from build123d import *

# Parameters (mm, degrees)
F0_R     = 6.35
F1_DEPTH = 10.16
F2_R     = 6.3201010277
F3_DEPTH = 12.7
F5_DEPTH = 10.16
F6_R     = 6.3201010277
F6_R_2   = 3.556
F7_DEPTH = 12.7


with BuildPart() as f1:
    # F0 (on Front) → F1 (new body)
    with BuildSketch(Plane.XZ):
        Circle(F0_R)
        with BuildLine():
            ThreePointArc((4.4769727705, 0.5322471811), (4.500611291, 0.2665900542), (4.5085, 0))
            ThreePointArc((4.5085, 0), (4.5084696907, -0.0165317216), (4.5083787633, -0.0330632208))
            ThreePointArc((4.5083787633, -0.0330632208), (4.4974064508, -0.3160814229), (4.4686849298, -0.597852196))
            ThreePointArc((4.4686849298, -0.597852196), (4.4223275509, -0.8772635196), (4.3585172655, -1.1532126849))
            ThreePointArc((4.3585172655, -1.1532126849), (4.2775059036, -1.4246106466), (4.1796131802, -1.6903863208))
            ThreePointArc((4.1796131802, -1.6903863208), (4.0652254331, -1.9494908126), (3.9347940983, -2.2009015547))
            ThreePointArc((3.9347940983, -2.2009015547), (3.788833929, -2.4436263439), (3.627920963, -2.6767072564))
            ThreePointArc((3.627920963, -2.6767072564), (3.4526902504, -2.8992244281), (3.2638333469, -3.1102996856))
            ThreePointArc((3.2638333469, -3.1102996856), (3.0620955841, -3.3091000111), (2.8482731291, -3.4948408307))
            ThreePointArc((2.8482731291, -3.4948408307), (2.6232098413, -3.6667891102), (2.3877939426, -3.8242662482))
            ThreePointArc((2.3877939426, -3.8242662482), (2.1429545122, -3.9666507546), (1.8896578193, -4.0933807025))
            ThreePointArc((1.8896578193, -4.0933807025), (1.6289035103, -4.203955947), (1.3617206633, -4.2979400979))
            ThreePointArc((1.3617206633, -4.2979400979), (1.089163727, -4.3749622428), (0.812308359, -4.4347184104))
            ThreePointArc((0.812308359, -4.4347184104), (0.5322471811, -4.4769727705), (0.2500854667, -4.5015585645))
            ThreePointArc((0.2500854667, -4.5015585645), (-0.0330632208, -4.5083787633), (-0.3160814229, -4.4974064508))
            ThreePointArc((-0.3160814229, -4.4974064508), (-0.597852196, -4.4686849298), (-0.8772635196, -4.4223275509))
            ThreePointArc((-0.8772635196, -4.4223275509), (-1.1532126849, -4.3585172655), (-1.4246106466, -4.2775059036))
            ThreePointArc((-1.4246106466, -4.2775059036), (-1.6903863208, -4.1796131802), (-1.9494908126, -4.0652254331))
            ThreePointArc((-1.9494908126, -4.0652254331), (-2.2009015547, -3.9347940983), (-2.4436263439, -3.788833929))
            ThreePointArc((-2.4436263439, -3.788833929), (-2.6767072564, -3.627920963), (-2.8992244281, -3.4526902504))
            ThreePointArc((-2.8992244281, -3.4526902504), (-3.1102996856, -3.2638333469), (-3.3091000111, -3.0620955841))
            ThreePointArc((-3.3091000111, -3.0620955841), (-3.4948408307, -2.8482731291), (-3.6667891102, -2.6232098413))
            ThreePointArc((-3.6667891102, -2.6232098413), (-3.8242662482, -2.3877939426), (-3.9666507546, -2.1429545122))
            ThreePointArc((-3.9666507546, -2.1429545122), (-4.0933807025, -1.8896578193), (-4.203955947, -1.6289035103))
            ThreePointArc((-4.203955947, -1.6289035103), (-4.2979400979, -1.3617206633), (-4.3749622428, -1.089163727))
            ThreePointArc((-4.3749622428, -1.089163727), (-4.4347184104, -0.812308359), (-4.4769727705, -0.5322471811))
            ThreePointArc((-4.4769727705, -0.5322471811), (-4.5015585645, -0.2500854667), (-4.5083787633, 0.0330632208))
            ThreePointArc((-4.5083787633, 0.0330632208), (-4.4974064508, 0.3160814229), (-4.4686849298, 0.597852196))
            ThreePointArc((-4.4686849298, 0.597852196), (-4.4223275509, 0.8772635196), (-4.3585172655, 1.1532126849))
            ThreePointArc((-4.3585172655, 1.1532126849), (-4.2775059036, 1.4246106466), (-4.1796131802, 1.6903863208))
            ThreePointArc((-4.1796131802, 1.6903863208), (-4.0652254331, 1.9494908126), (-3.9347940983, 2.2009015547))
            ThreePointArc((-3.9347940983, 2.2009015547), (-3.788833929, 2.4436263439), (-3.627920963, 2.6767072564))
            ThreePointArc((-3.627920963, 2.6767072564), (-3.4526902504, 2.8992244281), (-3.2638333469, 3.1102996856))
            ThreePointArc((-3.2638333469, 3.1102996856), (-3.0620955841, 3.3091000111), (-2.8482731291, 3.4948408307))
            ThreePointArc((-2.8482731291, 3.4948408307), (-2.6232098413, 3.6667891102), (-2.3877939426, 3.8242662482))
            ThreePointArc((-2.3877939426, 3.8242662482), (-2.1429545122, 3.9666507546), (-1.8896578193, 4.0933807025))
            ThreePointArc((-1.8896578193, 4.0933807025), (-1.6289035103, 4.203955947), (-1.3617206633, 4.2979400979))
            ThreePointArc((-1.3617206633, 4.2979400979), (-1.089163727, 4.3749622428), (-0.812308359, 4.4347184104))
            ThreePointArc((-0.812308359, 4.4347184104), (-0.5322471811, 4.4769727705), (-0.2500854667, 4.5015585645))
            ThreePointArc((-0.2500854667, 4.5015585645), (0.0330632208, 4.5083787633), (0.3160814229, 4.4974064508))
            ThreePointArc((0.3160814229, 4.4974064508), (0.597852196, 4.4686849298), (0.8772635196, 4.4223275509))
            ThreePointArc((0.8772635196, 4.4223275509), (1.1532126849, 4.3585172655), (1.4246106466, 4.2775059036))
            ThreePointArc((1.4246106466, 4.2775059036), (1.6903863208, 4.1796131802), (1.9494908126, 4.0652254331))
            ThreePointArc((1.9494908126, 4.0652254331), (2.2009015547, 3.9347940983), (2.4436263439, 3.788833929))
            ThreePointArc((2.4436263439, 3.788833929), (2.6767072564, 3.627920963), (2.8992244281, 3.4526902504))
            ThreePointArc((2.8992244281, 3.4526902504), (3.1102996856, 3.2638333469), (3.3091000111, 3.0620955841))
            ThreePointArc((3.3091000111, 3.0620955841), (3.4948408307, 2.8482731291), (3.6667891102, 2.6232098413))
            ThreePointArc((3.6667891102, 2.6232098413), (3.8242662482, 2.3877939426), (3.9666507546, 2.1429545122))
            ThreePointArc((3.9666507546, 2.1429545122), (4.0933807025, 1.8896578193), (4.203955947, 1.6289035103))
            ThreePointArc((4.203955947, 1.6289035103), (4.2979400979, 1.3617206633), (4.3749622428, 1.089163727))
            ThreePointArc((4.3749622428, 1.089163727), (4.4347184104, 0.812308359), (4.4769727705, 0.5322471811))
        make_face(mode=Mode.SUBTRACT)
    extrude(amount=F1_DEPTH)

    # F2 (on Front) → F3 (join)
    with BuildSketch(Plane.XZ):
        Circle(F2_R)
    extrude(amount=-F3_DEPTH)

    # F4 (on face) → F5 (cut)
    with BuildSketch(Plane(origin=(0, 12.7, 0), x_dir=(-1, 0, 0), z_dir=(0, 1, 0))):
        with BuildLine():
            ThreePointArc((-2.6027254946, 2.032), (-1.0744776445, -3.1222911125), (3.302, 0))
            ThreePointArc((3.302, 0), (3.1222911125, 1.0744776445), (2.6027254946, 2.032))
            Line((2.6027254946, 2.032), (-2.6027254946, 2.032))
        make_face()
    extrude(amount=-F5_DEPTH, mode=Mode.SUBTRACT)

    # F6 (on face) → F7 (join)
    with BuildSketch(Plane(origin=(0, 12.7, 0), x_dir=(-1, 0, 0), z_dir=(0, 1, 0))):
        Circle(F6_R)
        Circle(F6_R_2, mode=Mode.SUBTRACT)
        with BuildLine():
            Line((-2.6027254946, 2.032), (2.6027254946, 2.032))
            ThreePointArc((2.6027254946, 2.032), (0, 3.302), (-2.6027254946, 2.032))
        make_face()
    extrude(amount=-F7_DEPTH)


solid = f1.part
Source: CAD feature listing. Evaluate the final solid. Frame: model axes, mm. A direction names the side the tool comes from. Give positions to 0.01 mm unless a question says otherwise; leave off trailing zeros. Write each loop counter-clockwise with the first axis right and the second up, starting at its lowest first coordinate (ties: lowest second). Pieces come first, ordered by that corner, then holes. Notation, with made-up numbers: M 23.5,61 L 32.5,61 A21 cw 32.5,91 Z; hole C -14.5,49 d10. An arc over 180 degrees is marked long. Return JSON: item names as keys, results as strings. Group by question number.
1) Pull-direction query (Z, two-part tool) for faces 1 (the face through (0, 0, 0)), 2 (the face through (-5.015, 6.261, -3.846)), 3 (the face through (3, -10.16, -4)); classes: pulls with the +Z half, pulls with the -Z half, needs draft (parallel to the pull), parting line crosses it, or undercut.
2) Material intervals for line 1 along Z through (x, y) = (0, -1); line 2 along X through (y, z) = (7.5, 0); line 3 along Z through (x, y) = (0, 8.5), sorted ascending. Write a range as [from, to].
3) Pin query (flat end, axial travel): P1, Ø1.5, axis at x = 2, y = 4.5, coming from the -Z side; P2, Ø5, axis at x = -0.5, z = -2, coming from the +Y side; P3, Ø1.5, axis at y = 8.5, z = -3, coming from the -X side; P4, Ø1.5, axis at x = -1.5, z = -0.5, coming from the +Y side. Return the tip coordinate at first contact, or that it passes through.
4) Set-up query: faces 4 (the face through (0, 8, 2.032)), 5 (the face through (0, 12.7, 3)). Return all of +Z, -Z, +X, -X, +Y, -Y with unobstructed straight access to the full face (end or side cutting, diameter ignored); none if empty.
5) Cut plane B-B, the plane y = 5.5. Output: boundary loops of the cut face in (x, z), plus the area to 3 significant figures.
6) Cut plane C-C, the plane y = 1.75. Output: boundary loops of the cut face in (x, z), plus the area to 3 significant figures.
Recorded:
{
 "1": {"face 1": "undercut", "face 2": "parting line crosses it", "face 3": "needs draft"},
 "2": {"line 1": "z = [-6.35, -4.51], [4.51, 6.35]", "line 2": "x = [-6.32, -3.3], [3.3, 6.32]", "line 3": "z = [-6.32, -3.3], [2.03, 6.32]"},
 "3": {"P1": "stops at z = -6.2", "P2": "stops at y = 12.7", "P3": "stops at x = -5.91", "P4": "stops at y = 2.54"},
 "4": {"face 4": "+Y", "face 5": "+Z, -Z, +X, -X, +Y"},
 "5": {"outline": "C 0,0 d12.64; hole M -2.6,2.03 A3.3 ccw long 2.6,2.03 Z", "area": "95.8 mm²"},
 "6": {"outline": "C 0,0 d12.64", "area": "125 mm²"}
}
